Verification items for the finished model (mm, model axes). A direction names the side the tool comes from. Give positions to 0.01 mm unless a question says otherwise; leave off trailing zeros. Order: outer loops, then holes, each group sorted by start corner. A loop starts at its lowest first (then second) coordinate and runs counter-clockwise, first axis right, second up. Notation, with made-up numbers: (-17, 88.25) -> (40, 88.25) arc R22 ccw to (40, 94.25) -> close; hole circle Ø9 at (-16, -30). An arc over 180 degrees is marked (long way). Write each question's results on one line, items separated by ' | '. Start each with the question number.
1. Cross-section at C-C, the plane x = 0. Enter the section's corners in (y, z), then the cut area to 3 significant figures.
2. Material ranges on L1, parallel to Z at x = 38, y = 3.5; L2, parallel to Y at x = -44, z = -18; L3, parallel to X at y = 17, z = -13.5, recorded low to high. Write a range as from..to.
3. Depth check by flat-ended pin: pin 1 Ø4 at (x, y) = (-13.5, 4) entering from -Z; pin 2 Ø5 at (x, y) = (2, 19) entering from -Z; pin 3 Ø18 at (x, z) = (-25.5, 24) entering from +Y. Enter the tip coordinate at first touch or a pass-through.
4. Set-up check for faces 5 (the face through (37, 8.8, -36)), 6 (the face through (-36, 8.8, 37)), 7 (the face through (-19, 30.3, -4)), 8 (the face through (47.95, 4.34, 47.79)), 9 (the face through (-15.12, 19.7, 11.59)): record each of +Z, -Z, +X, -X, +Y, -Y from which the full face is reachable in a straight line by a thin tool's end or side.
5. Cross-section at A-A, the plane x = 43.5. Enter the section's corners in (y, z), then the cut area to 3 significant figures.
6. Cross-section at B-B, the plane y = 14. Enter the section's corners in (x, z).
7. Mould release check, pull along Z, two halves, no side actions. Record for faces 1 (the face through (50.8, 4, -30)), 2 (the face through (0.419, 8.593, 31.755)), 3 (the face through (38.377, 4.462, -36.085)), 4 (the face through (30, 4, -50.8)): +Z half, -Z half, draft (parallel to the pull), parting line (faces both ways), or undercut.
8. Cross-section at D-D, the plane z = -43.5. Enter the section's corners in (x, y).
Autodesk Inventor part; units mm, degrees
ref_plane "YZ Plane" through (0, 0, 0) normal (1, 0, 0) x (0, 1, 0)
ref_plane "XZ Plane" through (0, 0, 0) normal (0, 1, 0) x (-1, 0, 0)
ref_plane "XY Plane" through (0, 0, 0) normal (0, 0, 1) x (1, 0, 0)
sketch "Sketch1" plane through (0, 0, 0) normal (0, 1, 0) x (-1, 0, 0)
  line L0 (40.8, 50.8) -> (-40.8, 50.8)
  line L1 (-50.8, 40.8) -> (-50.8, -40.8)
  line L2 (-40.8, -50.8) -> (40.8, -50.8)
  line L3 (50.8, -40.8) -> (50.8, 40.8)
  line L4 (50.8, 50.8) -> (-50.8, -50.8) construction
  line L5 (-50.8, 50.8) -> (50.8, -50.8) construction
  arc A0 (50.8, 40.8) -> (40.8, 50.8) centre (40.8, 40.8) ccw
  arc A1 (-40.8, 50.8) -> (-50.8, 40.8) centre (-40.8, 40.8) ccw
  arc A2 (-50.8, -40.8) -> (-40.8, -50.8) centre (-40.8, -40.8) ccw
  arc A3 (40.8, -50.8) -> (50.8, -40.8) centre (40.8, -40.8) ccw
  point P0 (0, 0)
  dimension "d0" = 101.6
  dimension "d1" = 101.6
  dimension "d2" = 10
extrude "Extrusion1" add sketch "Sketch1" along normal blind 8.8
sketch "Sketch2" plane through (0, 0, 0) normal (1, 0, 0) x (0, 1, 0)
  line L0 (8.8, 40.8) -> (8.8, -40.8)
  line L1 (8.8, 0) -> (30.3, 0)
  line L2 (30.3, 0) -> (30.3, -25.4)
  line L3 (30.3, -25.4) -> (8.8, -41.28)
  line L4 (8.8, 0) -> (8.8, -41.28)
  line L5 (-49.004, 0) -> (294.024, 0)
  point P0 (0, 0)
  dimension "d5" = 25.4
  dimension "d6" = 21.5
  dimension "d7" = 41.28
revolve "Revolution1" add sketch "Sketch2" angle 360 about axis through (0, -10, 0) along (0, 1, 0)
sketch "Sketch3" plane through (0, 30.3, 0) normal (0, 1, 0) x (1, 0, 0)
  circle A0 centre (0, 0) radius 41.28
  circle A1 centre (0, 0) radius 19.05
  line L0 (40.8, 50.8) -> (-40.8, 50.8)
  arc A2 (-19.05, 50.8) -> (19.05, 50.8) centre (0, 50.8) ccw
  line L1 (50.8, -40.8) -> (50.8, 40.8)
  arc A3 (50.8, 19.05) -> (50.8, -19.05) centre (50.8, 0) ccw
  line L2 (-40.8, -50.8) -> (40.8, -50.8)
  arc A4 (19.05, -50.8) -> (-19.05, -50.8) centre (0, -50.8) ccw
  line L3 (-50.8, 40.8) -> (-50.8, -40.8)
  arc A5 (-50.8, -19.05) -> (-50.8, 19.05) centre (-50.8, 0) ccw
  line L4 (-50.8, -19.05) -> (-50.8, 19.05)
  line L5 (-19.05, 50.8) -> (19.05, 50.8)
  line L6 (50.8, 19.05) -> (50.8, -19.05)
  line L7 (19.05, -50.8) -> (-19.05, -50.8)
  line L8 (-39.031, 39.031) -> (39.031, 39.031)
  line L9 (39.031, 39.031) -> (39.031, -39.031)
  line L10 (39.031, -39.031) -> (-39.031, -39.031)
  line L11 (-39.031, -39.031) -> (-39.031, 39.031)
  line L12 (-39.031, 39.031) -> (39.031, -39.031) construction
  line L13 (39.031, 39.031) -> (-39.031, -39.031) construction
  circle A6 centre (-39.031, 39.031) radius 3.0175
  circle A7 centre (39.031, 39.031) radius 3.0175
  circle A8 centre (39.031, -39.031) radius 3.0175
  circle A9 centre (-39.031, -39.031) radius 3.0175
  point P0 (50.8, 19.05)
  dimension "d9" = 38.1
  dimension "d10" = 78.062
  dimension "d11" = 78.062
  dimension "d12" = 6.035
extrude "Extrusion2" cut sketch "Sketch3" against normal through all contours A0 L9 | A0 L9 A3 L1 | L9 A0 A3 | A0 A3 L9 | L9 A3 A0 | A2 A0 L8 | A0 L8 A2 | A4 L10 A0 | A0 L10 A4 | L8 A0 | A0 L8 A2 L0 | A2 L8 A0 | L10 A4 L2 A0 | A0 L10 | A0 L10 A4 | A5 A0 L11 | A0 L11 A5 | A5 L11 A0 | L11 A0 | A0 L11 A5 L3 | A1
extrude "Extrusion3" cut sketch "Sketch3" against normal through all contours A7 L8 L9 | L9 L8 A7 | A8 L10 L9 | L9 L10 A8 | A6 L11 L8 | L8 L11 A6 | A9 L11 L10 | L10 L11 A9
sketch "Sketch4" plane through (0, 0, 0) normal (0, -1, 0) x (1, 0, 0)
  circle A0 centre (0, 0) radius 19.05
  dimension "d19" = 38.1
extrude "Extrusion4" add sketch "Sketch4" against normal up to surface (8.8 mm away)
properties part number "WindTurbine"
Results below:
1) outline: (0, -31.75) -> (21.7, -31.75) -> (30.3, -25.4) -> (30.3, -19.05) -> (8.8, -19.05) -> (8.8, 19.05) -> (30.3, 19.05) -> (30.3, 25.4) -> (21.7, 31.75) -> (0, 31.75) -> close | area: 1,050 mm²
2) L1: z = -50.8..-41.87, -36.2..-14.11, 14.11..36.2, 41.87..50.8 | L2: y = 0..8.8 | L3: x = -32.53..-13.44, 13.44..32.53
3) pin 1: stops at z = -39.73 | pin 2: stops at z = -32.29 | pin 3: stops at y = 29.46
4) face 5: -Z, +X, +Y | face 6: +Z, -X, +Y | face 7: +Z, -Z, +X, -X, +Y | face 8: +Z, +X, +Y, -Y | face 9: +Y
5) outline: (0, -50.43) -> (8.8, -50.43) -> (8.8, -17.6) -> (0, -17.6) -> close; (0, 17.6) -> (8.8, 17.6) -> (8.8, 50.43) -> (0, 50.43) -> close | area: 578 mm²
6) outline: (-35.62, -11.52) arc R37.44 ccw to (-11.52, -35.62) arc R19.05 cw to (11.52, -35.62) arc R37.44 ccw to (35.62, -11.52) arc R19.05 cw to (35.62, 11.52) arc R37.44 ccw to (11.52, 35.62) arc R19.05 cw to (-11.52, 35.62) arc R37.44 ccw to (-35.62, 11.52) arc R19.05 cw to start; hole circle Ø38.1 at (0, 0)
7) face 1: draft | face 2: +Z half | face 3: undercut | face 4: -Z half
8) outline: (-50.43, 0) -> (-17.6, 0) -> (-17.6, 8.8) -> (-50.43, 8.8) -> close; (17.6, 0) -> (50.43, 0) -> (50.43, 8.8) -> (17.6, 8.8) -> close
